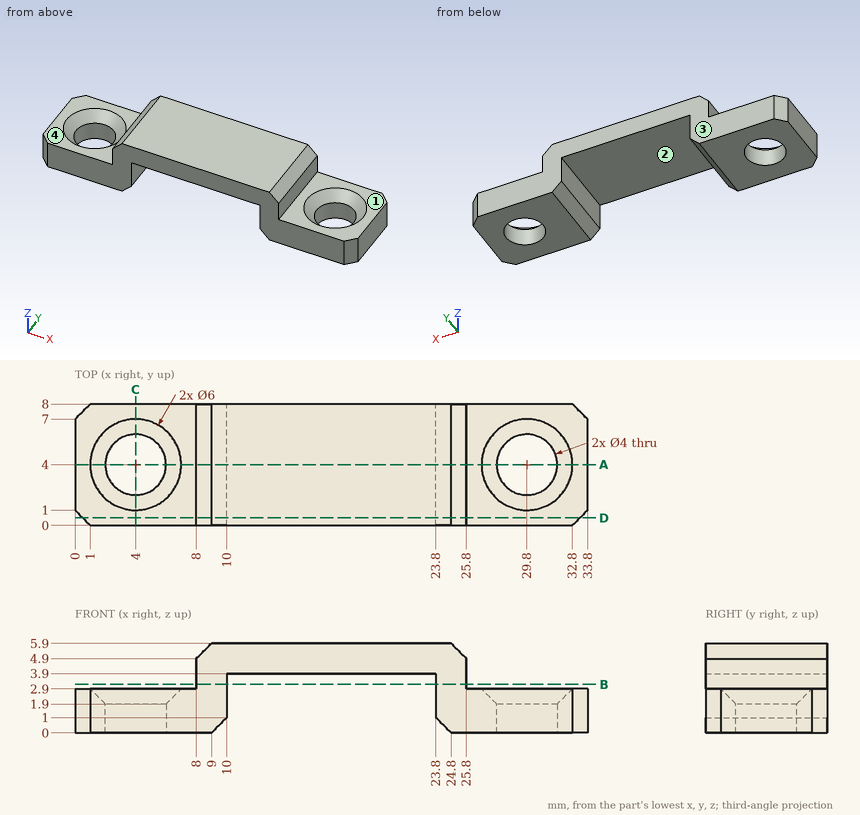
Answer from the drawing. Dimensions are ordinates in mm from the lowest x, y and z of the part. A direction names the side the tool comes from. Coordinates: 2 decimals unless noted, no trailing zeros. Write each loop counter-clockwise with the first axis right and the second up, starting at its lowest first coordinate (ties: lowest second). Pieces come first, ordered by that corner, then holes. Notation, with made-up numbers: M -28,76.5 L 18,76.5 A20 cw 18,93.5 Z; hole C 44,8.5 d2. An arc over 180 degrees is marked long. Use one line per item in the form item = value. Start each with the question number.
1. Each of these flat-tipped pins is pushed along its axis until it touches: P1, Ø1.5, axis at x = 14, z = 3.5, coming from the -Y side; P2, Ø2, axis at x = 27.5, y = 1, coming from the +Z side; P3, Ø1, axis at y = 3.5, z = 4, coming from the +X side; P4, Ø2, axis at y = 3, z = 4.5, coming from the -X side. Where does it stop, or does it pass through?
2. A tool of negligible diameter and unlimited length cuts with its end or side. For the marked faces 3 and 4, from which of +Z, -Z, +X, -X, +Y, -Y can it reach the whole face along a straight path? Write none if from no direction.
3. The part is cut by section D-D (y = 0.5). Give the vertices of the cut face in (x, z).
4. Straight lines are drawn through the part: probe 1 along Y at (x, z) = (29.8, 0.5); probe 2 along X at (y, z) = (1.75, 1.35); probe 3 along X at (y, z) = (7.5, 3.6). For each, find the intervals that lie inside material, in ascending order. Write a range as from..to.
5. The part is cut by section C-C (x = 4). Give the vertices of the cut face in (y, z).
6. The mould has two halves that part along X. Classify the marked faces 1 and 2: released by +X, released by -X, zero draft, split by the parting line, or undercut.
7. The part is cut by section B-B (z = 3.2). Give the vertices of the cut face in (x, y), plus the area to 3 significant figures.
8. The part is cut by section A-A (y = 4). Give the vertices of the cut face in (x, z).
Evaluation:
q1.P1 = 0
q1.P2 = 2.9
q1.P3 = 25.8
q1.P4 = 8
q2.face_3 = +Z, -Z, +X, -X, +Y
q2.face_4 = +Z, -X, +Y, -Y
q3.outline = M 0.5,0 L 9,0 L 10,1 L 10,3.9 L 23.8,3.9 L 23.8,1 L 24.8,0 L 33.3,0 L 33.3,2.9 L 25.8,2.9 L 25.8,4.9 L 24.8,5.9 L 9,5.9 L 8,4.9 L 8,2.9 L 0.5,2.9 Z
q4.probe_1 = 0..2, 6..8
q4.probe_2 = 0..10, 23.8..33.8
q4.probe_3 = 8..10, 23.8..25.8
q5.outline = M 0,0 L 2,0 L 2,1.9 L 1,2.9 L 0,2.9 Z; M 6,0 L 8,0 L 8,2.9 L 7,2.9 L 6,1.9 Z
q6.face_1 = zero draft
q6.face_2 = undercut
q7.outline = M 8,0 L 10,0 L 10,8 L 8,8 Z; M 23.8,0 L 25.8,0 L 25.8,8 L 23.8,8 Z
q7.area = 32.0 mm^2
q8.outline = M 0,0 L 2,0 L 2,1.9 L 1,2.9 L 0,2.9 Z; M 6,0 L 9,0 L 10,1 L 10,3.9 L 23.8,3.9 L 23.8,1 L 24.8,0 L 27.8,0 L 27.8,1.9 L 26.8,2.9 L 25.8,2.9 L 25.8,4.9 L 24.8,5.9 L 9,5.9 L 8,4.9 L 8,2.9 L 7,2.9 L 6,1.9 Z; M 31.8,0 L 33.8,0 L 33.8,2.9 L 32.8,2.9 L 31.8,1.9 Z
